from build123d import *

# Parameters (mm, degrees)
SKETCH_1_W                 = 15
SKETCH_1_H                 = 15
EXTRUDE_1_DEPTH            = 1.6
SKETCH_2_W                 = 10.960360983
SKETCH_2_H                 = 13.870606726
EXTRUDE_2_DEPTH            = 2.4
SKETCH_3_R                 = 0.3
CUT_EXTRUDE_1_DEPTH        = 2.4
PATTERN_LINEAR_1_COUNT     = 4
PATTERN_LINEAR_1_PITCH     = 2.54
PATTERN_LINEAR_1_COL_COUNT = 3
PATTERN_LINEAR_1_COL_PITCH = 2.54
CUT_EXTRUDE_2_DEPTH        = 0.01
CUT_EXTRUDE_3_DEPTH        = 0.01


with BuildPart() as part:
    # 草图1 → 凸台-拉伸1 (new body)
    with BuildSketch(Plane.XY):
        with Locations((7.5, 7.5)):
            Rectangle(SKETCH_1_W, SKETCH_1_H)
    extrude(amount=EXTRUDE_1_DEPTH)

    # 草图2 → 凸台-拉伸2 (add)
    with BuildSketch(Plane.XY.offset(1.6)):
        with Locations((7.453060553, 7.593878895)):
            Rectangle(SKETCH_2_W, SKETCH_2_H)
    extrude(amount=EXTRUDE_2_DEPTH)

    # 草图3 → 切除-拉伸1 (cut)
    with BuildSketch(Plane.XY.offset(1.6)):
        with Locations((1.15, 8.77)):
            Circle(SKETCH_3_R)
        with Locations((13.85, 8.77)):
            Circle(SKETCH_3_R)
    cut_extrude_1 = extrude(amount=-CUT_EXTRUDE_1_DEPTH, mode=Mode.SUBTRACT)

    # 阵列(线性)1: 切除-拉伸1 ×4
    with Locations(*[(0, -i * PATTERN_LINEAR_1_PITCH, 0) for i in range(1, PATTERN_LINEAR_1_COUNT)]):
        add(cut_extrude_1, mode=Mode.SUBTRACT)

    # 阵列(线性)1 col: 切除-拉伸1 ×3
    with Locations(*[(0, i * PATTERN_LINEAR_1_COL_PITCH, 0) for i in range(1, PATTERN_LINEAR_1_COL_COUNT)]):
        add(cut_extrude_1, mode=Mode.SUBTRACT)

    # 草图4 → 切除-拉伸2 (cut)
    with BuildSketch(Plane.XY.offset(4)):
        Polygon((10.539329223, 8.779099943), (10.539329223, 9.356105561), (12.417225748, 8.544402706), (10.539329223, 7.747506957), (10.539329223, 8.309705469), (4.272912987, 8.309705469), (4.272912987, 8.779099943), align=None)
    extrude(amount=-CUT_EXTRUDE_2_DEPTH, mode=Mode.SUBTRACT)

    # 草图5 → 切除-拉伸3 (cut)
    with BuildSketch(Plane.XY.offset(4)):
        with BuildLine():
            Line((11.417194479, 6.135405226), (11.641792388, 6.652462011))
            add(Edge.make_bspline(
                [(11.641792388, 6.652462011), (11.644459763, 6.65915976), (11.650338175, 6.673920386), (11.659052259, 6.698612128), (11.668619361, 6.727827369), (11.678458783, 6.760197023), (11.688890182, 6.792254636), (11.696772433, 6.821510802), (11.70401352, 6.845628042), (11.711125127, 6.871472603), (11.717769102, 6.901008766), (11.720240181, 6.924455008), (11.721474297, 6.936164633)],
                knots=[0, 0, 0, 0, 0.732180493, 1.613593324, 2.658872914, 3.854365511, 5.049858108, 6.082130019, 6.931166509, 7.607179292, 8.804966943, 10, 10, 10, 10], degree=3))
            Line((11.721474297, 6.936164633), (11.727603675, 6.986513092))
            Line((11.727603675, 6.986513092), (11.763066503, 6.992204657))
            Line((11.763066503, 6.992204657), (11.810350273, 6.743964863))
            add(Edge.make_bspline(
                [(11.810350273, 6.743964863), (11.803983049, 6.737631034), (11.792553049, 6.726260986), (11.777524458, 6.70884618), (11.763839933, 6.690929745), (11.750533347, 6.674158962), (11.738681861, 6.654023987), (11.727167788, 6.630404394), (11.713111944, 6.598523577), (11.70330589, 6.574415593), (11.697832412, 6.560959159)],
                knots=[0, 0, 0, 0, 0.993153163, 1.782839525, 2.541730564, 3.487713786, 4.146615727, 5.1212284, 6.393146485, 8, 8, 8, 8], degree=3))
            Line((11.697832412, 6.560959159), (11.458348872, 6.020260488))
            Line((11.458348872, 6.020260488), (11.756937125, 5.263720162))
            Line((11.756937125, 5.263720162), (11.816041838, 5.110047909))
            add(Edge.make_bspline(
                [(11.816041838, 5.110047909), (11.822079493, 5.096645389), (11.83288347, 5.072662481), (11.839984094, 5.042737639), (11.842976482, 5.023548034), (11.84296091, 5.013580004), (11.842191359, 5.006194655), (11.83795984, 5.000752614), (11.831545964, 4.998931147), (11.823968923, 4.993934019), (11.812279554, 5.002811857), (11.800976383, 5.014822536), (11.789795068, 5.028797256), (11.782777893, 5.036658786), (11.78057901, 5.039122253)],
                knots=[0, 0, 0, 0, 2.761412339, 4.941361911, 5.773257577, 6.405449525, 6.825913753, 7.139309286, 7.63100465, 8.075064367, 8.689683572, 10.011329248, 11.37683553, 12, 12, 12, 12], degree=3))
            Line((11.78057901, 5.039122253), (11.706588666, 5.103918531))
            add(Edge.make_bspline(
                [(11.706588666, 5.103918531), (11.700534721, 5.10864155), (11.689838198, 5.116986501), (11.676902014, 5.128864442), (11.668284845, 5.13690868), (11.662006372, 5.144967182), (11.663920439, 5.158199661), (11.663417087, 5.177036268), (11.664666192, 5.203655954), (11.661208157, 5.223194895), (11.659304896, 5.2339489)],
                knots=[0, 0, 0, 0, 1.23478745, 2.181706523, 2.812113369, 3.150477244, 3.760922406, 4.816942161, 6.248082283, 8, 8, 8, 8], degree=3))
            add(Edge.make_bspline(
                [(11.659304896, 5.2339489), (11.657570283, 5.243875719), (11.654377363, 5.262148127), (11.650117136, 5.28526259), (11.645361423, 5.305687518), (11.637884912, 5.326783626), (11.62842129, 5.355050264), (11.616354369, 5.387606437), (11.604632167, 5.419985798), (11.594840708, 5.447418485), (11.588025611, 5.467332719), (11.584154921, 5.478105212), (11.582687675, 5.482188694)],
                knots=[0, 0, 0, 0, 1.161118987, 2.137284709, 2.708267813, 3.575038829, 4.713036419, 6.143931784, 7.57482715, 8.681074464, 9.500040603, 10, 10, 10, 10], degree=3))
            Line((11.582687675, 5.482188694), (11.411065101, 5.916498881))
            Line((11.411065101, 5.916498881), (11.127362479, 5.2339489))
            Line((11.127362479, 5.2339489), (11.056436823, 5.071520392))
            add(Edge.make_bspline(
                [(11.056436823, 5.071520392), (11.05092025, 5.059923819), (11.040956646, 5.038978994), (11.027354455, 5.015348737), (11.016079719, 5.003114277), (11.011484356, 4.997021281), (11.004967483, 4.995661847), (11.003967513, 4.998937252), (11.003461488, 5.000594736)],
                knots=[0, 0, 0, 0, 2.381178734, 4.300699059, 5.010137615, 5.450112729, 5.721735305, 6, 6, 6, 6], degree=3))
            add(Edge.make_bspline(
                [(11.003461488, 5.000594736), (11.00235785, 5.001407174), (10.999053439, 5.003839699), (10.996910869, 5.011909178), (10.99504437, 5.022224411), (10.99599754, 5.033010837), (10.996542411, 5.043928598), (10.996917787, 5.0559064), (10.997475336, 5.07136957), (10.997383003, 5.082756589), (10.99733211, 5.0890329)],
                knots=[0, 0, 0, 0, 0.356334141, 1.066903249, 2.083622437, 3.166508591, 3.901872409, 4.984758563, 6.338055839, 8, 8, 8, 8], degree=3))
            Line((10.99733211, 5.0890329), (11.003461488, 5.207242326))
            add(Edge.make_bspline(
                [(11.003461488, 5.207242326), (11.003934057, 5.21659073), (11.004762277, 5.232974646), (11.007181535, 5.254267464), (11.008840176, 5.269124933), (11.012439148, 5.28195374), (11.023092765, 5.294221944), (11.037370069, 5.309576468), (11.05273668, 5.325448758), (11.065473263, 5.341432509), (11.075914366, 5.358198204), (11.086335771, 5.37372244), (11.096619807, 5.390411315), (11.105496545, 5.409732657), (11.116850923, 5.43433534), (11.129168728, 5.463048743), (11.141556256, 5.491950012), (11.152595687, 5.517741604), (11.16110265, 5.538779801), (11.166589578, 5.550938225), (11.168954684, 5.556179038)],
                knots=[0, 0, 0, 0, 1.283891209, 2.250134334, 2.938194825, 3.337125035, 4.054003749, 5.116665614, 6.235914532, 7.077065651, 7.915591523, 8.942962049, 9.643436631, 10.601555545, 11.855913542, 13.362341093, 14.887150874, 16.17010505, 17.211235183, 18, 18, 18, 18], degree=3))
            Line((11.168954684, 5.556179038), (11.36684602, 6.025952053))
            Line((11.36684602, 6.025952053), (11.14224811, 6.637576379))
            add(Edge.make_bspline(
                [(11.14224811, 6.637576379), (11.134802276, 6.653919815), (11.118638723, 6.689398443), (11.098117731, 6.734589073), (11.080824683, 6.771330602), (11.069237657, 6.795692229), (11.058270064, 6.815063097), (11.044964524, 6.835312795), (11.028432624, 6.859216492), (11.015814861, 6.87863072), (11.009153053, 6.888880863)],
                knots=[0, 0, 0, 0, 1.512108789, 3.282513405, 4.178459187, 4.931286787, 5.553090324, 6.050678811, 6.970815613, 8, 8, 8, 8], degree=3))
            Line((11.009153053, 6.888880863), (10.982884292, 6.924343691))
            Line((10.982884292, 6.924343691), (10.99733211, 6.968562772))
            Line((10.99733211, 6.968562772), (11.172019373, 6.906831183))
            add(Edge.make_bspline(
                [(11.172019373, 6.906831183), (11.172798131, 6.895160011), (11.174219289, 6.87386124), (11.175579615, 6.842681643), (11.179648195, 6.810360509), (11.185071037, 6.779955978), (11.192270701, 6.750508012), (11.200401611, 6.723903561), (11.209803376, 6.693508399), (11.217725107, 6.672414865), (11.22193002, 6.661218265)],
                knots=[0, 0, 0, 0, 1.113815777, 2.032607081, 2.970224408, 4.213083212, 4.971379877, 5.85514338, 6.861494526, 8, 8, 8, 8], degree=3))
            Line((11.22193002, 6.661218265), (11.417194479, 6.135405226))
        make_face()
    extrude(amount=-CUT_EXTRUDE_3_DEPTH, mode=Mode.SUBTRACT)


solid = part.part
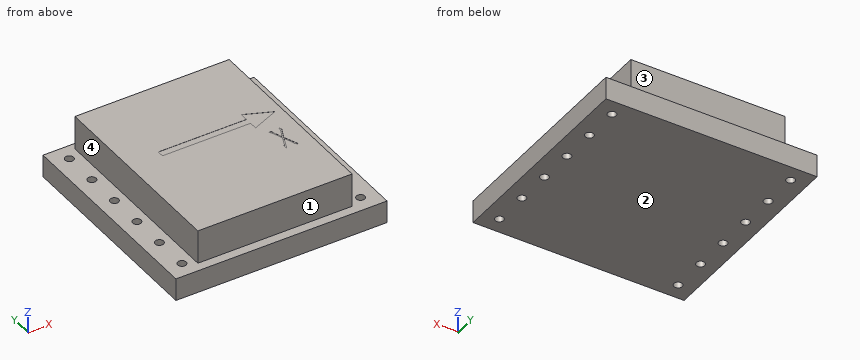
Read the model definition and answer for the solid it produces. Units are mm, in the model's axes. Face numbers are marked on the shaded views. A direction names the side the tool comes from. Coordinates: 2 decimals unless noted, no trailing zeros. Loops run counter-clockwise (first coordinate to the right, second up) from the corner with the lowest first, then second, coordinate; pieces in that order, holes last. Notation, with made-up numbers: (8.5, -16.75) -> (42.5, -16.75) arc R11 cw to (42.5, -6.75) -> close; hole circle Ø3 at (23, 66.5). An arc over 180 degrees is marked (long way). Answer in a Markdown table with one row per item.
Item 1: A cutting plane is placed at C-C on y = 2. Determine the outline of the cut face in (x, z), plus the area to 3 significant figures.
Returned:
| item | result |
|---|---|
| outline | (0, 0) -> (15, 0) -> (15, 1.6) -> (12.93, 1.6) -> (12.93, 4) -> (1.97, 4) -> (1.97, 1.6) -> (0, 1.6) -> close |
| area | 50.3 mm^2 |
Item 2: A cutting plane is placed at A-A on y = 3.69. Determine the outline of the cut face in (x, z).
Returned:
| item | result |
|---|---|
| outline | (0, 0) -> (0.85, 0) -> (0.85, 1.6) -> (0, 1.6) -> close; (1.45, 0) -> (13.55, 0) -> (13.55, 1.6) -> (12.93, 1.6) -> (12.93, 4) -> (1.97, 4) -> (1.97, 1.6) -> (1.45, 1.6) -> close; (14.15, 0) -> (15, 0) -> (15, 1.6) -> (14.15, 1.6) -> close |
Item 3: A cutting plane is placed at B-B on x = 1.15. Determine the outline of the cut face in (y, z), plus the area to 3 significant figures.
Returned:
| item | result |
|---|---|
| outline | (0, 0) -> (0.85, 0) -> (0.85, 1.6) -> (0, 1.6) -> close; (1.45, 0) -> (3.39, 0) -> (3.39, 1.6) -> (1.45, 1.6) -> close; (3.99, 0) -> (5.93, 0) -> (5.93, 1.6) -> (3.99, 1.6) -> close; (6.53, 0) -> (8.47, 0) -> (8.47, 1.6) -> (6.53, 1.6) -> close; (9.07, 0) -> (11.01, 0) -> (11.01, 1.6) -> (9.07, 1.6) -> close; (11.61, 0) -> (13.55, 0) -> (13.55, 1.6) -> (11.61, 1.6) -> close; (14.15, 0) -> (15, 0) -> (15, 1.6) -> (14.15, 1.6) -> close |
| area | 18.2 mm^2 |
Item 4: Straight lines are drawn through the part: line 1 along X through (y, z) = (11.31, 0.4); line 2 along X through (y, z) = (9, 1.45); line 3 along X through (y, z) = (8.75, 2.95). For each, find the intervals that lie inside material, in ascending order. Write a range as [from, to].
Returned:
| item | result |
|---|---|
| line 1 | x = [0, 0.85], [1.45, 13.55], [14.15, 15] |
| line 2 | x = [0, 0.96], [1.34, 13.66], [14.04, 15] |
| line 3 | x = [1.97, 12.93] |
Item 5: For the marked faces 1, 2, 3 and 4, determine the directions among +Z, -Z, +X, -X, +Y, -Y from which every point of the face is accessible in a straight line to the end or side of a thin tool.
Returned:
| item | result |
|---|---|
| face 1 | +Z, +X, -X, -Y |
| face 2 | -Z, +X, -X, +Y, -Y |
| face 3 | +Z, +X, -X, +Y |
| face 4 | +Z, -X, +Y, -Y |
Item 6: Each of these flat-tipped pins is pushed along its axis until it touches: P1, Ø0.7, axis at x = 7.5, z = 3, coming from the -Y side; P2, Ø0.7, axis at y = 5.5, z = 2.5, coming from the -X side; P3, Ø0.7, axis at y = 5, z = 3, coming from the +X side. Where does it stop, or does it pass through?
Returned:
| item | result |
|---|---|
| P1 | stops at y = 0.66 |
| P2 | stops at x = 1.97 |
| P3 | stops at x = 12.93 |
